Read the model definition and answer for the solid it produces. Units are mm, in the model's axes. Face numbers are marked on the shaded views. A direction names the side the tool comes from. Give positions to 0.01 mm unless a question says otherwise; leave off trailing zeros. Loops run counter-clockwise (first coordinate to the right, second up) from the corner with the lowest first, then second, coordinate; pieces in that order, holes last. Notation, with made-up numbers: (-39.5, -2) -> (-8.5, -2) arc R21 ccw to (-8.5, 26) -> close; hole circle Ø3 at (16.25, 82). An arc over 180 degrees is marked (long way). Write each question's results on one line, items separated by ' | '. Start each with the question number.
Item 1: Section A-A on x = 14.5 is taken. Write down the section's boundary in (y, z).
Item 2: Each of these flat-tipped pins is pushed along its axis until it touches: P1, Ø2, axis at y = 4, z = -4, coming from the +X side; P2, Ø8, axis at x = 11, z = -11.5, coming from the +Y side; P3, Ø1, axis at x = 11.5, y = 3.5, coming from the -Z side. Where does it stop, or does it pass through?
Item 3: Find the intervals of material crossed by line 1 (X direction, y = 2.8, z = 0); line 2 (X direction, y = 1.55, z = 0); line 3 (Y direction, x = 45, z = -12.5), in increasing order.
Item 4: Which of the six approach directions +Z, -Z, +X, -X, +Y, -Y give full straight-line access (tool end or side, diameter ignored) to the marked faces 1, 2 and 3?
Item 5: Section B-B on z = -7.9 is taken. Write down the section's boundary in (x, y), and give its area (3 significant figures).
Item 6: Section D-D on x = -14.5 is taken. Write down the section's boundary in (y, z), and give its area (3 significant figures).
Item 7: Section C-C on y = 7 is taken. Write down the section's boundary in (x, z), and give its area (3 significant figures).
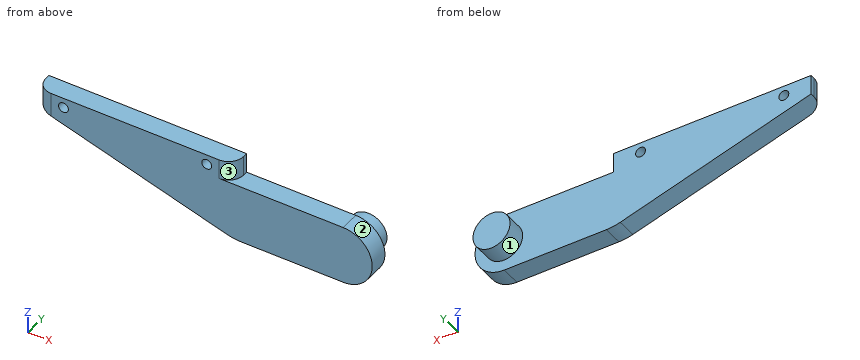
```python
from build123d import *

# Parameters (mm, degrees)
BOSS_EXTRUDE2_DEPTH = 4
SKETCH4_R           = 3.746181505
BOSS_EXTRUDE3_DEPTH = 4
SKETCH5_R           = 1
CUT_EXTRUDE1_DEPTH  = 9
FILLET1_R           = 10
FILLET3_R           = 3


with BuildPart() as part:
    # Sketch1 → Boss-Extrude2 (new body)
    with BuildSketch(Plane(origin=(0, 0, 0), x_dir=(1, 0, 0), z_dir=(0, 1, 0))):
        with BuildLine():
            Line((-20, 2), (20, 13.8))
            Line((20, 13.8), (42.1, 13.8))
            ThreePointArc((42.1, 13.8), (48, 7.9), (42.1, 2))
            Line((42.1, 2), (20, 2))
            Line((20, 2), (20, -2))
            Line((20, -2), (-20, -2))
            Line((-20, -2), (-20, 2))
        make_face()
    extrude(amount=BOSS_EXTRUDE2_DEPTH)

    # Sketch4 → Boss-Extrude3 (add)
    with BuildSketch(Plane(origin=(0, 4, 0), x_dir=(-1, 0, 0), z_dir=(0, -1, 0))):
        with Locations((-42.1, 7.9)):
            Circle(SKETCH4_R)
    extrude(amount=-BOSS_EXTRUDE3_DEPTH)

    # Sketch5 → Cut-Extrude1 (cut, through all)
    with BuildSketch(Plane(origin=(0, 0, 0), x_dir=(-1, 0, 0), z_dir=(0, -1, 0))):
        with Locations((14.5, 0)):
            Circle(SKETCH5_R)
        with Locations((-14.5, 0)):
            Circle(SKETCH5_R)
    extrude(amount=-CUT_EXTRUDE1_DEPTH, mode=Mode.SUBTRACT)

    # Fillet1
    fillet1_edges = [part.edges().sort_by_distance(p)[0] for p in [
        (20, 2, -13.8),
    ]]
    fillet(fillet1_edges, radius=FILLET1_R)

    # Fillet3
    fillet3_edges = [part.edges().sort_by_distance(p)[0] for p in [
        (20, 0, 0),
        (-20, 0, 0),
    ]]
    fillet(fillet3_edges, radius=FILLET3_R)


solid = part.part
```
Findings:
1) outline: (0, -12.18) -> (4, -12.18) -> (4, -1) -> (0, -1) -> close; (0, 1) -> (4, 1) -> (4, 2) -> (0, 2) -> close
2) P1: x = 47.24 | P2: y = 4 | P3: z = -11.44
3) line 1: -19.99 to -15.5, -13.5 to 13.5, 15.5 to 19.99 | line 2: -19.63 to -15.5, -13.5 to 13.5, 15.5 to 19.63 | line 3: 0 to 4
4) face 1: +Y | face 2: +X, +Y, -Y | face 3: +Z, +X, -Y
5) outline: (0, 0) -> (48, 0) -> (48, 4) -> (45.85, 4) -> (45.85, 8) -> (38.35, 8) -> (38.35, 4) -> (0, 4) -> close | area: 222 mm2
6) outline: (0, -3.62) -> (4, -3.62) -> (4, -1) -> (0, -1) -> close; (0, 1) -> (4, 1) -> (4, 2) -> (0, 2) -> close | area: 14.5 mm2
7) outline: circle Ø7.49 at (42.1, -7.9) | area: 44.1 mm2
